Model file for the job. Use its own axes, mm. Coordinates: 2 decimals unless noted, no trailing zeros. Write each loop counter-clockwise with the first axis right and the second up, starting at its lowest first coordinate (ties: lowest second). Pieces come first, ordered by that corner, then holes. Notation, with made-up numbers: M 80,77 L 122,77 A21 ccw 122,81 Z; hole C 82.5,-5 d3. An arc over 180 degrees is marked long. Use CSV: the item, a comma, the result in double quotes. Start each with the question number.
from build123d import *

# Parameters (mm, degrees)
SKETCH_1_W          = 10
SKETCH_1_H          = 20
SKETCH_1_R          = 3
EXTRUDE_1_DEPTH     = 10
SKETCH_2_R          = 1.65
CUT_EXTRUDE_1_DEPTH = 18.320508076
SKETCH_3_W          = 12.852703923
SKETCH_3_H          = 20.2795508
CUT_EXTRUDE_2_DEPTH = 16
FILLET_1_R          = 3


with BuildPart() as part:
    # 草圖1 → 填料-伸長1 (new body)
    with BuildSketch(Plane.XY):
        Rectangle(SKETCH_1_W, SKETCH_1_H)
        Circle(SKETCH_1_R, mode=Mode.SUBTRACT)
    extrude(amount=EXTRUDE_1_DEPTH)

    # 草圖2 → 除料-伸長1 (cut, through all)
    with BuildSketch(Plane.ZY.offset(5)):
        with Locations((5, 7)):
            Circle(SKETCH_2_R)
        with Locations((5, -7)):
            Circle(SKETCH_2_R)
    extrude(amount=-CUT_EXTRUDE_1_DEPTH, mode=Mode.SUBTRACT)

    # 草圖3 → 除料-伸長2 (cut, through all)
    with BuildSketch(Plane.XY.offset(10)):
        with Locations((6.426351961, -0.1397754)):
            Rectangle(SKETCH_3_W, SKETCH_3_H)
    extrude(amount=-CUT_EXTRUDE_2_DEPTH, mode=Mode.SUBTRACT)

    # 圓角1
    fillet_1_edges = [part.edges().sort_by_distance(p)[0] for p in [
        (-2.5, 10, 0),
        (-2.5, 10, 10),
        (-2.5, -10, 0),
        (-2.5, -10, 10),
    ]]
    fillet(fillet_1_edges, radius=FILLET_1_R)


solid = part.part
1) Band-saw the part on C-C on y = -7.5. List the corners of the cut face in (x, z), then the cut area to 3 significant figures.
2) Band-saw the part on A-A on z = 5. List the corners of the cut face in (x, y), then the cut area to 3 significant figures.
3) Drop a flat-ended pin along its axis: P1, Ø2, axis at y = -7, z = 5, coming from the +X side (1 decimal). Give the stop position or say it passes through.
4) Band-saw the part on D-D on x = -3.65. List the corners of the cut face in (y, z).
5) Band-saw the part on B-B on x = -2. List the corners of the cut face in (y, z).
6) Two-plate mould, pull along Y, no slides. Class faces 1 (the face through (-4, 0, 0)), 2 (the face through (-2.47, -9.14, 9.1)), 3 (the face through (-2.54, -8, 3.69)), 4 (the face through (-2.54, 6, 3.69)): pulls with the +Y half, pulls with the -Y half, needs draft (parallel to the pull), parting line crosses it, or undercut.
7) Wall check: L1, parallel to Y at x = -3.35, z = 5; L2, parallel to Y at x = -1.1, z = 5; L3, parallel to Y at x = -0.5, z = 6.5. Give the ranges that are in metal, low to high. Write a range as [from, to].
Findings below:
1,outline,"M -5,0.04 L 0,0.04 L 0,3.43 L -5,3.43 Z; M -5,6.57 L 0,6.57 L 0,9.96 L -5,9.96 Z"
1,area,"33.9 mm2"
2,outline,"M -5,-10 L 0,-10 L 0,-8.65 L -5,-8.65 Z; M -5,-5.35 L 0,-5.35 L 0,-3 A3 cw 0,3 L 0,5.35 L -5,5.35 Z; M -5,8.65 L 0,8.65 L 0,10 L -5,10 Z"
2,area,"52.9 mm2"
3,P1,"passes through"
4,outline,"M -10,3 A3 ccw -7,0 L 7,0 A3 ccw 10,3 L 10,7 A3 ccw 7,10 L -7,10 A3 ccw -10,7 Z; hole C -7,5 d3.3; hole C 7,5 d3.3"
5,outline,"M -10,3 A3 ccw -7,0 L -2.24,0 L -2.24,10 L -7,10 A3 ccw -10,7 Z; M 2.24,0 L 7,0 A3 ccw 10,3 L 10,7 A3 ccw 7,10 L 2.24,10 Z; hole C -7,5 d3.3; hole C 7,5 d3.3"
6,face 1,"needs draft"
6,face 2,"pulls with the -Y half"
6,face 3,"undercut"
6,face 4,"undercut"
7,L1,"y = [-10, -8.65], [-5.35, 5.35], [8.65, 10]"
7,L2,"y = [-10, -8.65], [-5.35, -2.79], [2.79, 5.35], [8.65, 10]"
7,L3,"y = [-10, -7.69], [-6.31, -2.96], [2.96, 6.31], [7.69, 10]"
